```python
from build123d import *

# Parameters (mm, degrees)
EXTRUDE_1_DEPTH     = 3
SKETCH_2_R          = 17.5
CUT_EXTRUDE_1_DEPTH = 142.453172464


with BuildPart() as part:
    # 草图1 → 凸台-拉伸1 (new body)
    with BuildSketch(Plane.XY):
        Polygon((-75, 100), (-75, 97), (-97, 97), (-97, 75), (-100, 75), (-100, 25), (-97, 25), (-97, 3), (-75, 3), (-75, 0), (-25, 0), (-25, 3), (-3, 3), (-3, 25), (0, 25), (0, 75), (-3, 75), (-3, 97), (-25, 97), (-25, 100), align=None)
    extrude(amount=EXTRUDE_1_DEPTH)

    # 草图2 → 切除-拉伸1 (cut, through all)
    with BuildSketch(Plane(origin=(0, 0, 0), x_dir=(-1, 0, 0), z_dir=(0, 0, -1))):
        with Locations((50, 50)):
            Circle(SKETCH_2_R)
    extrude(amount=-CUT_EXTRUDE_1_DEPTH, mode=Mode.SUBTRACT)


solid = part.part
```
Model file for the job. Use its own axes, mm. A direction names the side the tool comes from. Round coordinates to 2 decimals unless told otherwise and drop trailing zeros. Order: outer loops, then holes, each group sorted by start corner. A loop starts at its lowest first (then second) coordinate and runs counter-clockwise, first axis right, second up. Notation, with made-up numbers: (41, 64.25) -> (99, 64.25) arc R21 ccw to (99, 80.25) -> close; hole circle Ø8 at (-14.5, 72). An arc over 180 degrees is marked (long way). Use one line per item in the form item = value.
Item 1: Cut at B-B, the plane x = -50. Write the cut outline in (y, z), and give its area (3 significant figures).
Returned:
outline = (0, 0) -> (32.5, 0) -> (32.5, 3) -> (0, 3) -> close; (67.5, 0) -> (100, 0) -> (100, 3) -> (67.5, 3) -> close
area = 195 mm^2
Item 2: Cut at C-C, the plane y = 38.5. Write the cut outline in (x, z).
Returned:
outline = (-100, 0) -> (-63.19, 0) -> (-63.19, 3) -> (-100, 3) -> close; (-36.81, 0) -> (0, 0) -> (0, 3) -> (-36.81, 3) -> close
Item 3: Flat gauge pins, fed straight in: pin 1 Ø0.9 at (y, z) = (1.5, 2) entering from +X; pin 2 Ø1.5 at (x, z) = (-24.5, 1) entering from +Y; pin 3 Ø1.5 at (y, z) = (99, 1.5) entering from -X; pin 4 Ø0.9 at (x, z) = (-13, 1) entering from +Y. Where does each tip first touch, or does it go through?
Returned:
pin_1 = -25
pin_2 = 100
pin_3 = -75
pin_4 = 97
Item 4: Tool access for faces 1 (the face through (-100, 50, 1)), 2 (the face through (-25, 98, 1)), 3 (the face through (-25, 1, 1)), 4 (the face through (-97, 86, 1)), 5 (the face through (-99, 25, 1)): list every direction of +Z, -Z, +X, -X, +Y, -Y with a clear straight run to the whole face (end or side of a thin tool).
Returned:
face_1 = +Z, -Z, -X, +Y, -Y
face_2 = +Z, -Z, +X, +Y
face_3 = +Z, -Z, +X, -Y
face_4 = +Z, -Z, -X, +Y
face_5 = +Z, -Z, -X, -Y
Item 5: Cut at D-D, the plane y = 19.5. Write the cut outline in (x, z), and give its area (3 significant figures).
Returned:
outline = (-97, 0) -> (-3, 0) -> (-3, 3) -> (-97, 3) -> close
area = 282 mm^2
Item 6: Pull direction X, two halves, no side cores. Call faces 6 (the face through (-97, 14, 1)), 7 (the face through (-14, 3, 1)), 8 (the face through (-66.69, 55.26, 1.48)), 9 (the face through (0, 50, 1)): released by +X, released by -X, zero draft, split by the parting line, or undercut.
Returned:
face_6 = released by -X
face_7 = zero draft
face_8 = undercut
face_9 = released by +X
Item 7: Drill centre lines: line 1 (Y direction, x = -50, z = 2.3); line 2 (X direction, y = 15, z = 1.6); line 3 (X direction, y = 61, z = 1.5). Where is each one in solid material? Low to high.
Returned:
line_1 = 0 to 32.5, 67.5 to 100
line_2 = -97 to -3
line_3 = -100 to -63.61, -36.39 to 0
Item 8: Cut at A-A, the plane z = 0.45. Write the cut outline in (x, y), and give its area (3 significant figures).
Returned:
outline = (-100, 25) -> (-97, 25) -> (-97, 3) -> (-75, 3) -> (-75, 0) -> (-25, 0) -> (-25, 3) -> (-3, 3) -> (-3, 25) -> (0, 25) -> (0, 75) -> (-3, 75) -> (-3, 97) -> (-25, 97) -> (-25, 100) -> (-75, 100) -> (-75, 97) -> (-97, 97) -> (-97, 75) -> (-100, 75) -> close; hole circle Ø35 at (-50, 50)
area = 8,470 mm^2
